Geometry check sheet. Reference: the model listing, model coordinates, mm. A direction names the side the tool comes from. Round coordinates to 2 decimals unless told otherwise and drop trailing zeros. Write each loop counter-clockwise with the first axis right and the second up, starting at its lowest first coordinate (ties: lowest second). Pieces come first, ordered by that corner, then holes. Notation, with made-up numbers: (20.25, 27.25) -> (45.25, 27.25) arc R8 cw to (45.25, 37.25) -> close; hole circle Ø11 at (84.5, 11). An arc over 180 degrees is marked (long way). One line per question, with ' | ' between items.
```python
from build123d import *

# Parameters (mm, degrees)
F0_W     = 6
F0_H     = 0.3
F1_DEPTH = 7
F2_R     = 18
F3_DEPTH = 2
F4_R     = 2


# Not quite as in the source:
# - a feature names something its author has since deleted; it is built from what else it names


with BuildPart() as f1:
    # F0 (on Top) → F1 (new body)
    with BuildSketch(Plane.XY):
        with BuildLine():
            ThreePointArc((3.5, -3), (0, -3.3086313325), (-3.5, -3))
            Line((-3.5, -3), (-3.5, -65))
            Line((-3.5, -65), (-23.5, -65))
            Line((-23.5, -65), (-23.5, -70))
            Line((-23.5, -70), (-17.5, -70))
            Line((-17.5, -70), (-3.6, -70))
            Line((-3.6, -70), (-3.6, -67))
            Line((-3.6, -67), (3.6, -67))
            Line((3.6, -67), (3.6, -70))
            Line((3.6, -70), (17.5, -70))
            Line((17.5, -70), (23.5, -70))
            Line((23.5, -70), (23.5, -65))
            Line((23.5, -65), (3.5, -65))
            Line((3.5, -65), (3.5, -3))
        make_face()
        with BuildLine():
            ThreePointArc((20, 16.6913686675), (-12.8452325787, 32.0210783843), (-3.5, -3))
            ThreePointArc((-3.5, -3), (0, -3.3086313325), (3.5, -3))
            ThreePointArc((3.5, -3), (15.3297097168, 3.8461360889), (20, 16.6913686675))
        make_face()
        with Locations((-20.5, -70.15)):
            Rectangle(F0_W, F0_H)
        with Locations((20.5, -70.15)):
            Rectangle(F0_W, F0_H)
    extrude(amount=F1_DEPTH)

    # F2 (on face) → F3 (cut)
    with BuildSketch(Plane.XY.offset(7)):
        with Locations((0, 16.6913686675)):
            Circle(F2_R)
        with BuildLine():
            Line((0, 6.7382790148), (-2.256068401, 6.7382790148))
            Line((-2.256068401, 6.7382790148), (-2.256068401, 15.3757622465))
            add(Edge.make_bspline(
                [(-2.256068401, 15.3757622465), (-2.3233316964, 16.8329796939), (-2.719622442, 19.6479913649), (-7.1642837958, 22.803266535), (-7.7653425934, 23.4845241077)],
                knots=[0, 0, 0, 0, 0.4646113757, 1, 1, 1, 1], degree=3))
            Line((-7.7653425934, 23.4845241077), (-8.7472228794, 22.3505439034))
            Line((-8.7472228794, 22.3505439034), (-9.4585691677, 26.2563616887))
            Line((-9.4585691677, 26.2563616887), (-5.635671728, 26.2563616887))
            Line((-5.635671728, 26.2563616887), (-6.6175520141, 25.1223814843))
            add(Edge.make_bspline(
                [(0, 16.6913686675), (-0.8485280711, 18.3885709355), (-2.8253206301, 21.3582120071), (-5.1400469891, 24.3331446203), (-6.6175520141, 25.1223814843)],
                knots=[0, 0, 0, 0, 0.5076375045, 1, 1, 1, 1], degree=3))
            add(Edge.make_bspline(
                [(0, 16.6913686675), (0.8485280711, 18.3885709355), (2.8253206301, 21.3582120071), (5.1400469891, 24.3331446203), (6.6175520141, 25.1223814843)],
                knots=[0, 0, 0, 0, 0.5076375045, 1, 1, 1, 1], degree=3))
            Line((6.6175520141, 25.1223814843), (5.635671728, 26.2563616887))
            Line((5.635671728, 26.2563616887), (9.4585691677, 26.2563616887))
            Line((9.4585691677, 26.2563616887), (8.7472228794, 22.3505439034))
            Line((8.7472228794, 22.3505439034), (7.7653425934, 23.4845241077))
            add(Edge.make_bspline(
                [(2.256068401, 15.3757622465), (2.3233316964, 16.8329796939), (2.719622442, 19.6479913649), (7.1642837958, 22.803266535), (7.7653425934, 23.4845241077)],
                knots=[0, 0, 0, 0, 0.4646113757, 1, 1, 1, 1], degree=3))
            Line((2.256068401, 15.3757622465), (2.256068401, 6.7382790148))
            Line((2.256068401, 6.7382790148), (0, 6.7382790148))
        make_face(mode=Mode.SUBTRACT)
    extrude(amount=-F3_DEPTH, mode=Mode.SUBTRACT)

    # F4
    f4_edges = [f1.edges().sort_by_distance(p)[0] for p in [
        (-3.5, -3, 3.5),
        (3.5, -3, 3.5),
        (23.5, -65, 3.5),
        (-23.5, -65, 3.5),
        (-3.5, -65, 3.5),
        (3.5, -65, 3.5),
        (-23.5, -70.3, 3.5),
        (23.5, -70.3, 3.5),
    ]]
    fillet(f4_edges, radius=F4_R)


solid = f1.part
```
(1) Material ranges on line 1 (Z direction, x = 5.5, y = 20.5); line 2 (X direction, y = -29.5, z = 4.5); line 3 (X direction, y = 17.5, z = 4.25), recorded low to high.
Resolved:
line 1: z = 0 to 5 | line 2: x = -3.5 to 3.5 | line 3: x = -19.98 to 19.98
(2) Sectioned sample at A-A on y = -20. Record the cut outline in (x, z).
Resolved:
outline: (-3.5, 0) -> (3.5, 0) -> (3.5, 7) -> (-3.5, 7) -> close
(3) Access from +Z, -Z, +X, -X, +Y, -Y to the whole of each face (thin tool, end or side, straight path). Record for faces 1 (the flat face through (3.6, -68, 3)), 2 (the cylindrical face through (3.93, -3.37, 3.55)), 3 (the flat face through (-20, -70.3, 3)), 4 (the flat face through (0, 6.738, 6)), 5 (the flat face through (-3.5, -33, 3)).
Resolved:
face 1: +Z, -Z, -Y | face 2: +Z, -Z, +X | face 3: +Z, -Z, +X, -X, -Y | face 4: +Z | face 5: +Z, -Z, -X
(4) Go/stop test with flat-tipped pins: pin 1 (0.6 mm diameter, centred on x = -7.5, z = 5.5, fed in from +Y); pin 2 (1 mm diameter, centred on y = -17.5, z = 1.5, fed in from -X); pin 3 (2 mm diameter, centred on x = 10, z = 5, fed in from +Y). Record where each tip stops, or that it passes through.
Resolved:
pin 1: stops at y = 35.35 | pin 2: stops at x = -3.5 | pin 3: stops at y = 34.55
(5) Draft check along X on faces 6 (the flat face through (-9.1, 24.28, 6.01)), 7 (the cylindrical face through (-22.93, -69.7, 3.55)), 8 (the flat face through (0, -24, 7)). Enter one of: +X half, -X half, draft (parallel to the pull), parting line (faces both ways), or undercut.
Resolved:
face 6: undercut | face 7: -X half | face 8: draft
